Work out the finished part from the listing and answer in its coordinate system (mm). A direction names the side the tool comes from. Give positions to 0.01 mm unless a question says otherwise; leave off trailing zeros. Order: outer loops, then holes, each group sorted by start corner. A loop starts at its lowest first (then second) coordinate and runs counter-clockwise, first axis right, second up.
```python
from build123d import *

# Parameters (mm, degrees)
SKETCH1_W           = 497
SKETCH1_H           = 176.5
BOSS_EXTRUDE1_DEPTH = 18
SKETCH5_R           = 2.5
CUT_EXTRUDE4_DEPTH  = 18
SKETCH6_R           = 5
CUT_EXTRUDE5_DEPTH  = 12


with BuildPart() as part:
    # Sketch1 → Boss-Extrude1 (new body)
    with BuildSketch(Plane.XY):
        with Locations((0, -302.75)):
            Rectangle(SKETCH1_W, SKETCH1_H)
    extrude(amount=BOSS_EXTRUDE1_DEPTH)

    # Sketch5 → Cut-Extrude4 (cut)
    with BuildSketch(Plane.XY.offset(18)):
        with Locations((64, -302.75)):
            Circle(SKETCH5_R)
        with Locations(Location((-64, -302.75, 0), (0, 0, 180))):
            Circle(SKETCH5_R)
    extrude(amount=-CUT_EXTRUDE4_DEPTH, mode=Mode.SUBTRACT)

    # Sketch6 → Cut-Extrude5 (cut)
    with BuildSketch(Plane(origin=(0, 0, 0), x_dir=(-1, 0, 0), z_dir=(0, 0, -1))):
        with Locations((224, -270.5)):
            Circle(SKETCH6_R)
        with Locations(Location((-224, -270.5, 0), (0, 0, 180))):
            Circle(SKETCH6_R)
        with Locations((224, -334.5)):
            Circle(SKETCH6_R)
        with Locations(Location((-224, -334.5, 0), (0, 0, 180))):
            Circle(SKETCH6_R)
    extrude(amount=-CUT_EXTRUDE5_DEPTH, mode=Mode.SUBTRACT)


solid = part.part
```
1. The part is cut by section A-A (y = -270.5). Write down the section's boundary in (x, z), then the cut area to 3 significant figures.
Findings below:
outline: (-248.5, 0) - (-229, 0) - (-229, 12) - (-219, 12) - (-219, 0) - (219, 0) - (219, 12) - (229, 12) - (229, 0) - (248.5, 0) - (248.5, 18) - (-248.5, 18) - close
area: 8,710 mm2
2. The mould has two halves that part along Y. Classify faces 3 (the face through (248.5, -304, 9)), 4 (the face through (-3, -214.5, 9)), 5 (the face through (-224, -270, 12)), 6 (the face through (224, -271, 12)): pulls with the +Y half, pulls with the -Y half, needs draft (parallel to the pull), parting line crosses it, or undercut.
Findings below:
face 3: needs draft
face 4: pulls with the +Y half
face 5: undercut
face 6: undercut
3. The part is cut by section B-B (x = -224). Write down the section's boundary in (y, z).
Findings below:
outline: (-391, 0) - (-339.5, 0) - (-339.5, 12) - (-329.5, 12) - (-329.5, 0) - (-275.5, 0) - (-275.5, 12) - (-265.5, 12) - (-265.5, 0) - (-214.5, 0) - (-214.5, 18) - (-391, 18) - close
4. Given P1, Ø4.5, axis at x = 64, y = -302.75, coming from the -Z side; P2, Ø3, axis at x = -224, y = -272.5, coming from the -Z side, each flat-ended and moving along its own axis, determine where each tip first touches the part or whether it passes through.
Findings below:
P1: passes through
P2: stops at z = 12
5. Which of the six approach directions +Z, -Z, +X, -X, +Y, -Y give full straight-line access (tool end or side, diameter ignored) to faces 1 (the face through (-3, -302, 0)), 2 (the face through (-224, -334, 12))?
Findings below:
face 1: -Z, +X, -X, +Y, -Y
face 2: -Z
6. Straight lines are drawn through the part: probe 1 along Y at (x, z) = (-224, 5.75); probe 2 along X at (y, z) = (-270.5, 7); probe 3 along X at (y, z) = (-302.75, 6.75). For each, find the intervals that lie inside material, in ascending order.
Findings below:
probe 1: y = -391 to -339.5, -329.5 to -275.5, -265.5 to -214.5
probe 2: x = -248.5 to -229, -219 to 219, 229 to 248.5
probe 3: x = -248.5 to -66.5, -61.5 to 61.5, 66.5 to 248.5
